from build123d import *

# Parameters (mm, degrees)
BOSS_EXTRUDE1_DEPTH = 3.175
SKETCH2_R           = 12.7
BOSS_EXTRUDE2_DEPTH = 254
BOSS_EXTRUDE3_START = 19.90327871
BOSS_EXTRUDE3_DEPTH = 19.90327871
SKETCH15_W          = 9.525
SKETCH15_H          = 155.575
CHAMFER1_SIZE       = 19.880208588
CHAMFER1_SIZE_2     = 9.525


with BuildPart() as part:
    # Sketch1 → Boss-Extrude1 (new, symmetric)
    with BuildSketch(Plane.XY):
        with BuildLine():
            Line((9.951639355, 67.400163523), (9.951639355, -67.400163523))
            ThreePointArc((9.951639355, -67.400163523), (0, -77.351802878), (-9.951639355, -67.400163523))
            Line((-9.951639355, -67.400163523), (-9.951639355, 67.400163523))
            ThreePointArc((-9.951639355, 67.400163523), (0, 77.351802878), (9.951639355, 67.400163523))
        make_face()
        with BuildLine():
            Line((3.601639355, 67.400163523), (3.601639355, -67.400163523))
            ThreePointArc((3.601639355, -67.400163523), (0, -71.001802878), (-3.601639355, -67.400163523))
            Line((-3.601639355, -67.400163523), (-3.601639355, 67.400163523))
            ThreePointArc((-3.601639355, 67.400163523), (0, 71.001802878), (3.601639355, 67.400163523))
        make_face(mode=Mode.SUBTRACT)
    extrude(amount=BOSS_EXTRUDE1_DEPTH, both=True)

    # Sketch2 → Boss-Extrude2 (add)
    with BuildSketch(Plane(origin=(9.951639355, 0, 0), x_dir=(0, 0, -1), z_dir=(1, 0, 0))):
        with Locations(Location((0, 0, 0), (0, 0, 104.477512186))):
            Circle(SKETCH2_R)
    extrude(amount=BOSS_EXTRUDE2_DEPTH)

    # Sketch5 → Boss-Extrude3 (add)
    with BuildSketch(Plane.ZY.offset(-9.951639355).offset(BOSS_EXTRUDE3_START)):
        with BuildLine():
            Line((-3.175, -12.296722124), (-3.175, 12.296722124))
            ThreePointArc((-3.175, 12.296722124), (-12.7, 0), (-3.175, -12.296722124))
        make_face()
        with BuildLine():
            Line((3.175, 12.296722124), (3.175, -12.296722124))
            ThreePointArc((3.175, -12.296722124), (12.7, 0), (3.175, 12.296722124))
        make_face()
    extrude(amount=-BOSS_EXTRUDE3_DEPTH)

    # Sketch15 → Cut-Revolve2 (revolve, cut)
    with BuildSketch(Plane.ZY.offset(9.951639355)):
        with Locations((-7.9375, 77.7875)):
            Rectangle(SKETCH15_W, SKETCH15_H)
    revolve(axis=Axis((-9.951639355, 0, -3.175), (0, 0, -1)), mode=Mode.SUBTRACT)

    # Chamfer1
    # the kernel refuses this chamfer: 19.880208588, 9.525 mm, written as the material it takes off along each edge
    with BuildSketch(Plane(origin=(-9.951639355, 0, 0), x_dir=(0, -0.003141587485879782, -0.9999950652018581), z_dir=(0, 0.9999950652018581, -0.003141587485879782))) as chamfer1_piece_1_section:
        Polygon((12.7, -CHAMFER1_SIZE), (12.7 - CHAMFER1_SIZE_2, 0), (12.7, 0), align=None)
    chamfer1_piece_1 = revolve(axis=Axis((-9.951639355, 0, 0), (-1, 0, 0)), revolution_arc=359.64, mode=Mode.PRIVATE)
    chamfer1_piece_1 = split(chamfer1_piece_1, bisect_by=Plane(origin=(-9.951639355, 0, 3.175), z_dir=(0, 0, 1)), keep=Keep.TOP, mode=Mode.PRIVATE)
    add(chamfer1_piece_1, mode=Mode.SUBTRACT)


solid = part.part
Work out the finished part from the listing and answer in its coordinate system (mm). A direction names the side the tool comes from. Coordinates: 2 decimals unless noted, no trailing zeros. Order: outer loops, then holes, each group sorted by start corner. A loop starts at its lowest first (then second) coordinate and runs counter-clockwise, first axis right, second up. Notation, with made-up numbers: (-17, 1) - (-2, 1) arc R29 ccw to (-2, 40) - close; hole circle Ø6 at (11.5, -22). An arc over 180 degrees is marked (long way). Put each result on its own line as item: value. Start each with the question number.
1) Find section D-D (x = 158). Give the vertices of the cut face in (y, z) (3 decimals).
2) Flat-ended cylindrical pins translate along their axes: pin 1 (3 mm diameter, centred on x = 65.5, z = 5, fed in from +Y); pin 2 (8 mm diameter, centred on x = 212.5, z = 3, fed in from -Y); pin 3 (5 mm diameter, centred on y = -32, z = -0.5, fed in from +X). Find the tip coordinate at first contact, or state that the pin passes through.
3) Find section C-C (x = 0). Give the vertices of the cut face in (y, z) (3 decimals).
4) Find section A-A (z = 0). Give the vertices of the cut face in (x, y).
5) Find section B-B (y = -19). Give the vertices of the cut face in (x, z) (3 decimals).
6) For faces 4 (the flat face through (0, 0, 3.175)), 5 (the flat face through (9.952, -39, 0)), 6 (the cylindrical face through (0, 71, 0)), 7 (the cylindrical face through (145.623, 0.172, -6.814)), determine the directions among +Z, -Z, +X, -X, +Y, -Y from which every point of the face is accessible in a straight line to the end or side of a thin tool.
7) For a pull along Y with two mould halves and no side action, classify faces 1 (the flat face through (9.952, 40, 0)), 2 (the cylindrical face through (-0.22, 77.35, 0.04)), 3 (the flat face through (-3.602, -1, 0)) as released by +Y, released by -Y, zero draft, split by the parting line, or undercut.
8) Find the intervals of material crossed by line 1 (X direction, y = -40, z = 0.25); line 2 (X direction, y = -2.5, z = 2.75); line 3 (Y direction, x = 27.5, z = -1), in increasing order. Write a range as from..to.
Results list:
1. outline: circle Ø25.4 at (0, 0)
2. pin 1: stops at y = 12.21
2. pin 2: stops at y = -12.7
2. pin 3: stops at x = 9.95
3. outline: (-77.352, -3.175) - (-71.002, -3.175) - (-71.002, 3.175) - (-77.352, 3.175) - close; (-7.281, 3.175) - (7.281, 3.175) arc R7.943 ccw to start; (71.002, -3.175) - (77.352, -3.175) - (77.352, 3.175) - (71.002, 3.175) - close
4. outline: (-9.95, -67.4) arc R9.95 ccw to (9.95, -67.4) - (9.95, -12.7) - (263.95, -12.7) - (263.95, 12.7) - (9.95, 12.7) - (9.95, 67.4) arc R9.95 ccw to (-9.95, 67.4) - close; hole (-3.6, -67.4) arc R3.6 ccw to (3.6, -67.4) - (3.6, 67.4) arc R3.6 ccw to (-3.6, 67.4) - close
5. outline: (-9.952, -3.175) - (-3.602, -3.175) - (-3.602, 3.175) - (-9.952, 3.175) - close; (3.602, -3.175) - (9.952, -3.175) - (9.952, 3.175) - (3.602, 3.175) - close
6. face 4: -Z
6. face 5: +Z, -Z, +X, -Y
6. face 6: +Z, -Z
6. face 7: -Z, -X
7. face 1: zero draft
7. face 2: released by +Y
7. face 3: undercut
8. line 1: x = -9.95..-3.6, 3.6..9.95
8. line 2: x = -9.95..-3.6, 3.6..263.95
8. line 3: y = -12.66..12.66
